The model under review builds one solid part; all positions refer to its coordinate system, in mm. Round coordinates to 2 decimals unless told otherwise and drop trailing zeros. Use one line per item in the form item = value.
Autodesk Inventor part; units mm, degrees
ref_plane "YZ Plane" through (0, 0, 0) normal (1, 0, 0) x (0, 1, 0)
ref_plane "XZ Plane" through (0, 0, 0) normal (0, 1, 0) x (-1, 0, 0)
ref_plane "XY Plane" through (0, 0, 0) normal (0, 0, 1) x (1, 0, 0)
sketch "Sketch1" plane through (0, 0, 0) normal (0, 1, 0) x (-1, 0, 0)
  circle A0 centre (0, 0) radius 2.1
  line L0 (10, 10) -> (-10, 10) construction
  line L1 (-10, 10) -> (-10, -10) construction
  line L2 (-10, -10) -> (10, -10) construction
  line L3 (10, -10) -> (10, 10) construction
  line L4 (10, 10) -> (-10, -10) construction
  line L5 (-10, 10) -> (10, -10) construction
  line L6 (8.2, 10) -> (8.2, -10) construction
  line L7 (3.9, 10) -> (3.9, -10) construction
  line L8 (8.2, 3.125) -> (8.2, -3.125) construction
  line L9 (10, 4.58) -> (10, -4.58) construction
  line L10 (8.2, 5.5) -> (8.2, -5.5) construction
  line L11 (3.3697, 4.4303) -> (4.4303, 3.3697) construction
  line L12 (10, 10) -> (10, 4.58)
  line L13 (10, 4.58) -> (8.545, 3.125)
  line L14 (8.545, 3.125) -> (8.2, 3.125)
  line L15 (8.2, 3.125) -> (8.2, 5.5)
  line L16 (14, 0) -> (-14, 0) construction
  line L17 (8.2, 5.5) -> (6.5607, 5.5)
  line L18 (6.5607, 5.5) -> (3.9, 2.8393)
  line L19 (3.9, 2.8393) -> (3.9, 0)
  line L20 (10, -10) -> (10, -4.58)
  line L21 (10, -4.58) -> (8.545, -3.125)
  line L22 (8.545, -3.125) -> (8.2, -3.125)
  line L23 (8.2, -3.125) -> (8.2, -5.5)
  line L24 (8.2, -5.5) -> (6.5607, -5.5)
  line L25 (6.5607, -5.5) -> (3.9, -2.8393)
  line L26 (3.9, -2.8393) -> (3.9, 0)
  line L27 (-10, 10) -> (-4.58, 10)
  line L28 (-4.58, 10) -> (-3.125, 8.545)
  line L29 (-3.125, 8.2) -> (-5.5, 8.2)
  line L30 (-5.5, 8.2) -> (-5.5, 6.5607)
  line L31 (-5.5, 6.5607) -> (-2.8393, 3.9)
  line L32 (-2.8393, 3.9) -> (0, 3.9)
  line L33 (2.8393, 3.9) -> (0, 3.9)
  line L34 (5.5, 6.5607) -> (2.8393, 3.9)
  line L35 (5.5, 8.2) -> (5.5, 6.5607)
  line L36 (3.125, 8.2) -> (5.5, 8.2)
  line L37 (3.125, 8.545) -> (3.125, 8.2)
  line L38 (4.58, 10) -> (3.125, 8.545)
  line L39 (-3.125, 8.545) -> (-3.125, 8.2)
  line L40 (10, 10) -> (4.58, 10)
  line L41 (-10, -10) -> (-10, -4.58)
  line L42 (-10, -4.58) -> (-8.545, -3.125)
  line L43 (-8.2, -3.125) -> (-8.2, -5.5)
  line L44 (-8.2, -5.5) -> (-6.5607, -5.5)
  line L45 (-6.5607, -5.5) -> (-3.9, -2.8393)
  line L46 (-3.9, -2.8393) -> (-3.9, 0)
  line L47 (-3.9, 2.8393) -> (-3.9, 0)
  line L48 (-6.5607, 5.5) -> (-3.9, 2.8393)
  line L49 (-8.2, 5.5) -> (-6.5607, 5.5)
  line L50 (-8.2, 3.125) -> (-8.2, 5.5)
  line L51 (-8.545, 3.125) -> (-8.2, 3.125)
  line L52 (-10, 4.58) -> (-8.545, 3.125)
  line L53 (-8.545, -3.125) -> (-8.2, -3.125)
  line L54 (-10, 10) -> (-10, 4.58)
  line L55 (10, -10) -> (4.58, -10) construction
  line L56 (4.58, -10) -> (3.125, -8.545) construction
  line L57 (3.125, -8.2) -> (5.5, -8.2) construction
  line L58 (5.5, -8.2) -> (5.5, -6.5607) construction
  line L59 (5.5, -6.5607) -> (2.8393, -3.9)
  line L60 (2.8393, -3.9) -> (0, -3.9)
  line L61 (-2.8393, -3.9) -> (0, -3.9)
  line L62 (-5.5, -6.5607) -> (-2.8393, -3.9)
  line L63 (-5.5, -8.2) -> (-5.5, -6.5607) construction
  line L64 (-3.125, -8.2) -> (-5.5, -8.2) construction
  line L65 (-3.125, -8.545) -> (-3.125, -8.2) construction
  line L66 (-4.58, -10) -> (-3.125, -8.545) construction
  line L67 (3.125, -8.545) -> (3.125, -8.2) construction
  line L68 (-10, -10) -> (-4.58, -10) construction
  line L69 (5.5, -6.5607) -> (6.2393, -7.3)
  line L70 (6.2393, -7.3) -> (8.2, -7.3)
  line L71 (0, -10) -> (0, -9) construction
  line L72 (-5.5, -6.5607) -> (-6.2393, -7.3)
  line L73 (-6.2393, -7.3) -> (-8.2, -7.3)
  line L74 (8.2, -7.3) -> (8.2, -10)
  line L75 (-8.2, -7.3) -> (-8.2, -10)
  circle A1 centre (0, -20) radius 2.1
  line L76 (10, -30) -> (10, -24.58)
  line L77 (10, -24.58) -> (8.545, -23.125)
  line L78 (8.545, -23.125) -> (8.2, -23.125)
  line L79 (8.2, -23.125) -> (8.2, -25.5)
  line L80 (8.2, -25.5) -> (6.5607, -25.5)
  line L81 (6.5607, -25.5) -> (3.9, -22.8393)
  line L82 (3.9, -22.8393) -> (3.9, -20)
  line L83 (10, -10) -> (10, -15.42)
  line L84 (10, -15.42) -> (8.545, -16.875)
  line L85 (8.2, -16.875) -> (8.2, -14.5)
  line L86 (8.2, -14.5) -> (6.5607, -14.5)
  line L87 (6.5607, -14.5) -> (3.9, -17.1607)
  line L88 (3.9, -17.1607) -> (3.9, -20)
  line L89 (-10, -30) -> (-4.58, -30)
  line L90 (-4.58, -30) -> (-3.125, -28.545)
  line L91 (-3.125, -28.2) -> (-5.5, -28.2)
  line L92 (-5.5, -28.2) -> (-5.5, -26.5607)
  line L93 (-5.5, -26.5607) -> (-2.8393, -23.9)
  line L94 (-2.8393, -23.9) -> (0, -23.9)
  line L95 (2.8393, -23.9) -> (0, -23.9)
  line L96 (5.5, -26.5607) -> (2.8393, -23.9)
  line L97 (5.5, -28.2) -> (5.5, -26.5607)
  line L98 (3.125, -28.2) -> (5.5, -28.2)
  line L99 (3.125, -28.545) -> (3.125, -28.2)
  line L100 (4.58, -30) -> (3.125, -28.545)
  line L101 (-3.125, -28.545) -> (-3.125, -28.2)
  line L102 (10, -30) -> (4.58, -30)
  line L103 (-10, -10) -> (-10, -15.42)
  line L104 (-10, -15.42) -> (-8.545, -16.875)
  line L105 (-8.2, -16.875) -> (-8.2, -14.5)
  line L106 (-8.2, -14.5) -> (-6.5607, -14.5)
  line L107 (-6.5607, -14.5) -> (-3.9, -17.1607)
  line L108 (-3.9, -17.1607) -> (-3.9, -20)
  line L109 (-3.9, -22.8393) -> (-3.9, -20)
  line L110 (-6.5607, -25.5) -> (-3.9, -22.8393)
  line L111 (-8.2, -25.5) -> (-6.5607, -25.5)
  line L112 (-8.2, -23.125) -> (-8.2, -25.5)
  line L113 (-8.545, -23.125) -> (-8.2, -23.125)
  line L114 (-10, -24.58) -> (-8.545, -23.125)
  line L115 (-8.545, -16.875) -> (-8.2, -16.875)
  line L116 (-10, -30) -> (-10, -24.58)
  line L117 (5.5, -13.4393) -> (2.8393, -16.1)
  line L118 (2.8393, -16.1) -> (0, -16.1)
  line L119 (-2.8393, -16.1) -> (0, -16.1)
  line L120 (-5.5, -13.4393) -> (-2.8393, -16.1)
  line L121 (5.5, -13.4393) -> (6.2393, -12.7)
  line L122 (6.2393, -12.7) -> (8.2, -12.7)
  line L123 (-5.5, -13.4393) -> (-6.2393, -12.7)
  line L124 (-6.2393, -12.7) -> (-8.2, -12.7)
  line L125 (8.2, -12.7) -> (8.2, -10)
  line L126 (-8.2, -12.7) -> (-8.2, -10)
  line L127 (8.545, -16.875) -> (8.2, -16.875)
  point P0 (10, 0)
  point P1 (8.2, 0)
  point P2 (3.9, 3.9)
  point P3 (-3.3697, 4.4303)
  point P4 (-4.4303, -3.3697)
  point P5 (3.3697, -4.4303)
  dimension "d0" = 4.2
  dimension "d1" = 20
  dimension "d2" = 20
  dimension "d3" = 1.8
  dimension "d4" = 4.3
  dimension "d5" = 6.25
  dimension "d6" = 9.16
  dimension "d7" = 11
  dimension "d8" = 1.5
  dimension "d9" = 45
  dimension "d12" = 360
  dimension "d17" = 1.8
  dimension "d18" = 1
extrude "Extrusion1" add sketch "Sketch1" along normal blind 600
ref_plane "Work Plane1" through (-2.8393, 0, 0) normal (0, 0, -1) x (-1, 0, 0)
ref_plane "Work Plane2" through (0, 0, 4.58) normal (1, 0, 0) x (0, 0, -1)
ref_plane "Work Plane3" through (0, 300, 0) normal (0, 1, 0) x (1, 0, 0)
ref_plane "Work Plane4" through (2.8393, 0, -20) normal (0, 0, 1) x (1, 0, 0)
properties part number "VSLOT 2020 Extrusion"
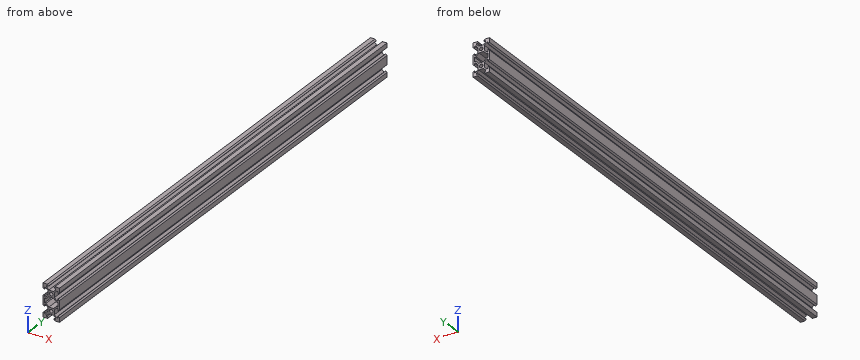
(1) Insertion check: P1, Ø6, axis at y = 293, z = -0.5, coming from the -X side; P2, Ø4.5, axis at y = 208, z = -19.5, coming from the -X side. Each pin has a flat end and moves straight along its axis. Give the tip position at first contact, or say it passes through.
Geometry results:
P1 = -8.92
P2 = -3.9
(2) To check wall thickness, follow L1, parallel to Z at x = 0, y = 276; L2, parallel to Z at x = 8, y = 148; L3, parallel to X at y = 544.5, z = 7. State the ranges of each line that lie inside material, in increasing order.
Geometry results:
L1 = -23.9 to -22.1, -17.9 to -16.1, -3.9 to -2.1, 2.1 to 3.9
L2 = -30 to -25.5, -14.5 to -12.7, -7.3 to -5.5, 5.5 to 10
L3 = -10 to -5.5, 5.5 to 10
(3) Add section A-A on y = 264. Count the separate pieces of the cut face and the enclosed holes in it, then the cut area to 3 significant figures.
Geometry results:
separate_pieces = 1
enclosed_holes = 3
area = 300 mm2
